Source: CAD feature listing. Evaluate the final solid. Frame: model axes, mm. Give positions to 0.01 mm unless a question says otherwise; leave off trailing zeros. Write each loop counter-clockwise with the first axis right and the second up, starting at its lowest first coordinate (ties: lowest second). Pieces come first, ordered by that corner, then holes. Notation, with made-up numbers: (-23.75, -38.75) -> (-18.75, -38.75) arc R24 cw to (-18.75, -7.75) -> close; hole circle Ø11 at (0, 34.25). An arc over 180 degrees is marked (long way). Write item = value, one per line.
from build123d import *

# Parameters (mm, degrees)
SKIZZE1_R                       = 5
AUFSATZ_LINEAR_AUSTRAGEN1_DEPTH = 335
SKIZZE2_R                       = 2.5
SCHNITT_LINEAR_AUSTRAGEN3_DEPTH = 17
SKIZZE3_R                       = 2.5
SCHNITT_LINEAR_AUSTRAGEN4_DEPTH = 17


with BuildPart() as part:
    # Skizze1 → Aufsatz-Linear austragen1 (new body)
    with BuildSketch(Plane.XY):
        Circle(SKIZZE1_R)
    extrude(amount=AUFSATZ_LINEAR_AUSTRAGEN1_DEPTH)

    # Skizze2 → Schnitt-Linear austragen3 (cut)
    with BuildSketch(Plane.XY):
        Circle(SKIZZE2_R)
    extrude(amount=SCHNITT_LINEAR_AUSTRAGEN3_DEPTH, mode=Mode.SUBTRACT)

    # Skizze3 → Schnitt-Linear austragen4 (cut)
    with BuildSketch(Plane.XY.offset(335)):
        Circle(SKIZZE3_R)
    extrude(amount=-SCHNITT_LINEAR_AUSTRAGEN4_DEPTH, mode=Mode.SUBTRACT)


solid = part.part
1) Cut plane A-A (x = 0). Return the cut outline in (y, z).
Computed:
outline = (-5, 0) -> (-2.5, 0) -> (-2.5, 17) -> (2.5, 17) -> (2.5, 0) -> (5, 0) -> (5, 335) -> (2.5, 335) -> (2.5, 318) -> (-2.5, 318) -> (-2.5, 335) -> (-5, 335) -> close
2) Material intervals for L1, parallel to Y at x = 0, z = 7.5; L2, parallel to X at y = -0.5, z = 99; L3, parallel to Z at x = 0.75, y = 0, sorted ascending.
Computed:
L1 = -5 to -2.5, 2.5 to 5
L2 = -4.97 to 4.97
L3 = 17 to 318
3) Contact query for flat-ended pins moving along their axis: pin 1 (2.5 mm diameter, centred on x = 0.5, y = 0.5, fed in from -Z); pin 2 (3 mm diameter, centred on y = -2.5, z = 243, fed in from +X); pin 3 (2.5 mm diameter, centred on x = 0.5, y = -0.5, fed in from +Z). Output: stop coordinate, or through.
Computed:
pin_1 = 17
pin_2 = 4.9
pin_3 = 318
4) Cut plane C-C (z = 210.5). Return the cut outline in (x, y).
Computed:
outline = circle Ø10 at (0, 0)
